CAD build for the part. Positions are in the model's coordinates, mm. A direction names the side the tool comes from. Give positions to 0.01 mm unless a question says otherwise; leave off trailing zeros. Order: outer loops, then holes, each group sorted by start corner. A loop starts at its lowest first (then second) coordinate and runs counter-clockwise, first axis right, second up.
Item 1: Band-saw the part on D-D on x = 254. Give the cut face in (y, z), plus the area to 3 significant figures.
Item 2: Two-plate mould, pull along Z, no slides. Class faces 1 (the flat face through (84, 10, -234.594)), 2 (the flat face through (147, 19.05, -245)), 3 (the flat face through (246.939, 9.658, -451.294)): released by +Z, released by -Z, zero draft, split by the parting line, or undercut.
Item 3: Flat gauge pins, fed straight in: P1, Ø15, axis at x = 160, z = -418.5, coming from the +Y side; P2, Ø10, axis at x = 65.5, y = 8.5, coming from the -Z side; P3, Ø1, axis at x = 235.5, y = 14, coming from the -Z side. Where does each tip first touch, or does it go through?
Item 4: Band-saw the part on A-A on z = -342.5. Give the cut face in (x, y), plus the area to 3 significant figures.
Item 5: Band-saw the part on C-C on z = -12.7. Give the cut face in (x, y).
Item 6: Which spindle directions (+Z, -Z, +X, -X, +Y, -Y) get a long thin tool onto all of the face, cutting with end or side? Do faces 4 (the flat face through (155.2, 12.7, -428.3)), 5 (the flat face through (147, 0, -245)), 6 (the flat face through (214, 10, -38.1)). Say none if no direction does.
Item 7: Wall check: L1, parallel to Z at x = 114.3, y = 5; L2, parallel to X at y = 7, z = -59 (3 decimals); L3, parallel to Z at x = 209, y = 7. Give the ranges that are in metal, low to high.
Item 8: Band-saw the part on B-B on x = 62. Give the cut face in (y, z).
```python
from build123d import *

# Parameters (mm, degrees)
SKETCH1_W                    = 298.45
SKETCH1_H                    = 482.6
BOSS_EXTRUDE1_DEPTH          = 19.05
F_1_2_0_5_DIAMETER_HOLE1_D   = 12.7
LPATTERN1_COUNT              = 4
LPATTERN1_PITCH              = 69.85
LPATTERN1_COUNT_DIR2         = 2
LPATTERN1_PITCH_DIR2         = 247.2944
F_3_8_0_375_DIAMETER_HOLE1_D = 9.525
SKETCH6_R                    = 25.4
CUT_EXTRUDE1_DEPTH           = 6.35
F_3_4_10_TAPPED_HOLE1_D      = 16.66748
SKETCH10_W                   = 92.075
SKETCH10_H                   = 196.4944
SKETCH10_H_2                 = 76.5556
CUT_EXTRUDE2_DEPTH           = 568.74824086
FILLET1_R                    = 12.7
CUT_EXTRUDE3_DEPTH           = 568.74824086
CUT_EXTRUDE4_DEPTH           = 568.74824086


with BuildPart() as part:
    # Sketch1 → Boss-Extrude1 (new body)
    with BuildSketch(Plane(origin=(0, 0, 0), x_dir=(1, 0, 0), z_dir=(0, 1, 0))):
        with Locations((149.225, 241.3)):
            Rectangle(SKETCH1_W, SKETCH1_H)
    extrude(amount=BOSS_EXTRUDE1_DEPTH)

    # 1/2 (0.5) Diameter Hole1 (through all)
    with Locations(Plane(origin=(0, 19.05, 0), x_dir=(1, 0, 0), z_dir=(0, 1, 0))):
        with Locations((44.45, 12.7)):
            f_1_2_0_5_diameter_hole1 = Hole(F_1_2_0_5_DIAMETER_HOLE1_D / 2)

    # LPattern1: 1_2 _0.5_ Diameter Hole1 4 × 2
    with Locations(*[(i * LPATTERN1_PITCH, 0, -j * LPATTERN1_PITCH_DIR2) for i in range(LPATTERN1_COUNT) for j in range(LPATTERN1_COUNT_DIR2) if (i, j) != (0, 0)]):
        add(f_1_2_0_5_diameter_hole1, mode=Mode.SUBTRACT)

    # 3/8 (0.375) Diameter Hole1 (through all)
    with Locations(Plane(origin=(0, 19.05, 0), x_dir=(1, 0, 0), z_dir=(0, 1, 0))):
        with Locations((284.1625, 400.05), (14.2875, 400.05)):
            Hole(F_3_8_0_375_DIAMETER_HOLE1_D / 2)

    # Sketch6 → Cut-Extrude1 (cut)
    with BuildSketch(Plane(origin=(0, 19.05, 0), x_dir=(1, 0, 0), z_dir=(0, 1, 0))):
        with Locations(Location((149.225, 422.275, 0), (0, 0, 270))):
            Circle(SKETCH6_R)
    extrude(amount=-CUT_EXTRUDE1_DEPTH, mode=Mode.SUBTRACT)

    # 3/4-10 Tapped Hole1 (through all)
    with Locations(Plane(origin=(0, 0, 0), x_dir=(-1, 0, 0), z_dir=(0, -1, 0))):
        with Locations((-149.225, 422.275)):
            Hole(F_3_4_10_TAPPED_HOLE1_D / 2)

    # Sketch10 → Cut-Extrude2 (cut, through all)
    with BuildSketch(Plane(origin=(0, 19.05, 0), x_dir=(1, 0, 0), z_dir=(0, 1, 0))):
        with Locations((84.1375, 136.3472)):
            Rectangle(SKETCH10_W, SKETCH10_H)
        with Locations((214.3125, 136.3472)):
            Rectangle(SKETCH10_W, SKETCH10_H)
        with Locations((84.1375, 323.6722)):
            Rectangle(SKETCH10_W, SKETCH10_H_2)
        with Locations((214.3125, 323.6722)):
            Rectangle(SKETCH10_W, SKETCH10_H_2)
    extrude(amount=-CUT_EXTRUDE2_DEPTH, mode=Mode.SUBTRACT)

    # Fillet1
    fillet1_edges = [part.edges().sort_by_distance(p)[0] for p in [
        (38.1, 9.525, -38.1),
        (38.1, 9.525, -234.5944),
        (130.175, 9.525, -234.5944),
        (130.175, 9.525, -38.1),
        (168.275, 9.525, -38.1),
        (168.275, 9.525, -234.5944),
        (260.35, 9.525, -234.5944),
        (260.35, 9.525, -38.1),
        (38.1, 9.525, -285.3944),
        (38.1, 9.525, -361.95),
        (130.175, 9.525, -361.95),
        (130.175, 9.525, -285.3944),
        (168.275, 9.525, -285.3944),
        (168.275, 9.525, -361.95),
        (260.35, 9.525, -361.95),
        (260.35, 9.525, -285.3944),
    ]]
    fillet(fillet1_edges, radius=FILLET1_R)

    # Sketch11 → Cut-Extrude3 (cut, through all)
    with BuildSketch(Plane(origin=(0, 19.05, 0), x_dir=(1, 0, 0), z_dir=(0, 1, 0))):
        Polygon((0, 482.6), (0, 419.1), (101.6, 482.6), align=None)
        Polygon((298.45, 482.6), (196.85, 482.6), (298.45, 419.1), align=None)
    extrude(amount=-CUT_EXTRUDE3_DEPTH, mode=Mode.SUBTRACT)

    # Sketch12 → Cut-Extrude4 (cut, through all)
    with BuildSketch(Plane(origin=(0, 19.05, 0), x_dir=(1, 0, 0), z_dir=(0, 1, 0))):
        with BuildLine():
            Line((50.8, 285.3944), (247.65, 285.3944))
            ThreePointArc((247.65, 285.3944), (256.630256121, 289.114143879), (260.35, 298.0944))
            Line((260.35, 298.0944), (260.35, 361.5944))
            ThreePointArc((260.35, 361.5944), (256.630256121, 370.574656121), (247.65, 374.2944))
            Line((247.65, 374.2944), (50.8, 374.2944))
            ThreePointArc((50.8, 374.2944), (41.819743879, 370.574656121), (38.1, 361.5944))
            Line((38.1, 361.5944), (38.1, 298.0944))
            ThreePointArc((38.1, 298.0944), (41.819743879, 289.114143879), (50.8, 285.3944))
        make_face()
    extrude(amount=-CUT_EXTRUDE4_DEPTH, mode=Mode.SUBTRACT)


solid = part.part
```
The answers:
1. outline: (0, -446.88) - (19.05, -446.88) - (19.05, -372.59) - (0, -372.59) - close; (0, -287.1) - (19.05, -287.1) - (19.05, -266.34) - (0, -266.34) - close; (0, -253.64) - (19.05, -253.64) - (19.05, -232.89) - (0, -232.89) - close; (0, -39.8) - (19.05, -39.8) - (19.05, -19.05) - (0, -19.05) - close; (0, -6.35) - (19.05, -6.35) - (19.05, 0) - (0, 0) - close
1. area: 2,720 mm2
2. face 1: undercut
2. face 2: zero draft
2. face 3: released by -Z
3. P1: stops at y = 12.7
3. P2: stops at z = -463.16
3. P3: stops at z = -458.76
4. outline: (0, 0) - (38.1, 0) - (38.1, 19.05) - (0, 19.05) - close; (260.35, 0) - (298.45, 0) - (298.45, 19.05) - (260.35, 19.05) - close
4. area: 1,450 mm2
5. outline: (0, 0) - (38.1, 0) - (38.1, 19.05) - (0, 19.05) - close; (50.8, 0) - (107.95, 0) - (107.95, 19.05) - (50.8, 19.05) - close; (120.65, 0) - (177.8, 0) - (177.8, 19.05) - (120.65, 19.05) - close; (190.5, 0) - (247.65, 0) - (247.65, 19.05) - (190.5, 19.05) - close; (260.35, 0) - (298.45, 0) - (298.45, 19.05) - (260.35, 19.05) - close
6. face 4: +Y
6. face 5: +Z, -Z, +X, -X, -Y
6. face 6: +Y, -Y
7. L1: z = -482.6 to -374.29, -285.39 to -266.34, -253.64 to -234.59, -38.1 to -19.05, -6.35 to 0
7. L2: x = 0 to 38.1, 130.175 to 168.275, 260.35 to 298.45
7. L3: z = -475.01 to -374.29, -285.39 to -234.59, -38.1 to 0
8. outline: (0, -457.85) - (19.05, -457.85) - (19.05, -374.29) - (0, -374.29) - close; (0, -285.39) - (19.05, -285.39) - (19.05, -234.59) - (0, -234.59) - close; (0, -38.1) - (19.05, -38.1) - (19.05, 0) - (0, 0) - close
